from build123d import *

# Parameters (mm, degrees)
F1_DEPTH = 13
F2_R     = 1.5
F3_DEPTH = 1
F4_R     = 1.5
F5_DEPTH = 1


with BuildPart() as f1:
    # F0 (on Right) → F1 (new body)
    with BuildSketch(Plane.YZ):
        Polygon((-7.5, -7), (-6.5, -7), (-6.5, 6), (7.5, 6), (7.5, 7), (-7.5, 7), align=None)
    extrude(amount=F1_DEPTH)

    # F2 (on face) → F3 (cut, through all)
    with BuildSketch(Plane.XY.offset(7)):
        with Locations((6.5, 0)):
            Circle(F2_R)
    extrude(amount=-F3_DEPTH, mode=Mode.SUBTRACT)

    # F4 (on face) → F5 (cut, through all)
    with BuildSketch(Plane.XZ.offset(7.5)):
        with Locations((6.5, 0.5)):
            Circle(F4_R)
    extrude(amount=-F5_DEPTH, mode=Mode.SUBTRACT)


solid = f1.part
Geometry: final body of the model. Coordinates: model frame, mm. A direction names the side the tool comes from. Give positions to 0.01 mm unless a question says otherwise; leave off trailing zeros. Order: outer loops, then holes, each group sorted by start corner. A loop starts at its lowest first (then second) coordinate and runs counter-clockwise, first axis right, second up. Notation, with made-up numbers: (39.5, -18.75) -> (48.5, -18.75) arc R24 cw to (48.5, 1.25) -> close; hole circle Ø10 at (-4.5, 9.5). An arc over 180 degrees is marked (long way). Write each question's results on one line, items separated by ' | '.
1) Cut plane B-B (x = 6.5). Output: boundary loops of the cut face in (y, z), and give its area (3 significant figures).
Geometry says:
outline: (-7.5, -7) -> (-6.5, -7) -> (-6.5, -1) -> (-7.5, -1) -> close; (-7.5, 2) -> (-6.5, 2) -> (-6.5, 6) -> (-1.5, 6) -> (-1.5, 7) -> (-7.5, 7) -> close; (1.5, 6) -> (7.5, 6) -> (7.5, 7) -> (1.5, 7) -> close | area: 22.0 mm²
2) Cut plane A-A (z = 0.5). Output: boundary loops of the cut face in (x, y), and give its area (3 significant figures).
Geometry says:
outline: (0, -7.5) -> (5, -7.5) -> (5, -6.5) -> (0, -6.5) -> close; (8, -7.5) -> (13, -7.5) -> (13, -6.5) -> (8, -6.5) -> close | area: 10.0 mm²
3) Line query: line 1 along Z through (x, y) = (6.5, -6.95); line 2 along Y through (x, z) = (6.5, 6.5); line 3 along Y through (x, z) = (10.25, -2.75). Output: solid intervals per line, ascending.
Geometry says:
line 1: z = -7 to -1, 2 to 7 | line 2: y = -7.5 to -1.5, 1.5 to 7.5 | line 3: y = -7.5 to -6.5
4) Set-up query: faces 1 (the face through (5, -7.01, 0.57)), 2 (the face through (6, -6.5, -2)). Return all of +Z, -Z, +X, -X, +Y, -Y with unobstructed straight access to the full face (end or side cutting, diameter ignored); none if empty.
Geometry says:
face 1: +Y, -Y | face 2: -Z, +X, -X, +Y
5) First-contact query: pin 1 Ø6.5 at (x, z) = (8, -3.5) entering from +Y; pin 2 Ø6 at (x, y) = (3, 4.5) entering from -Z. Flat tips, straight axial feed; report the tip coordinate or a pass-through.
Geometry says:
pin 1: stops at y = -6.5 | pin 2: stops at z = 6
6) Draft query along Y for faces 3 (the face through (6.4, 7.5, 6.5)), 4 (the face through (5, 0.07, 6.51)), 5 (the face through (0, -3.4, 6.3)). Return one class per face: released by +Y, released by -Y, zero draft, split by the parting line, or undercut.
Geometry says:
face 3: released by +Y | face 4: undercut | face 5: zero draft
7) Cut plane D-D (x = 11.5). Output: boundary loops of the cut face in (y, z).
Geometry says:
outline: (-7.5, -7) -> (-6.5, -7) -> (-6.5, 6) -> (7.5, 6) -> (7.5, 7) -> (-7.5, 7) -> close
8) Cut plane C-C (y = 0). Output: boundary loops of the cut face in (x, z).
Geometry says:
outline: (0, 6) -> (5, 6) -> (5, 7) -> (0, 7) -> close; (8, 6) -> (13, 6) -> (13, 7) -> (8, 7) -> close
